Autodesk Inventor part; units mm, degrees
ref_plane "YZ Plane" through (0, 0, 0) normal (1, 0, 0) x (0, 1, 0)
ref_plane "XZ Plane" through (0, 0, 0) normal (0, 1, 0) x (-1, 0, 0)
ref_plane "XY Plane" through (0, 0, 0) normal (0, 0, 1) x (1, 0, 0)
sketch "Sketch1" plane through (0, 0, 0) normal (0, 1, 0) x (-1, 0, 0)
  line L0 (0, 0) -> (-25, 0)
  line L1 (-25, 0) -> (-25, -14)
  line L2 (-25, -14) -> (0, -14)
  line L3 (0, -14) -> (0, 0)
  dimension "d0" = 25
  dimension "d1" = 14
extrude "Extrusion1" add sketch "Sketch1" along normal blind 14
sketch "Sketch2" plane through (0, 14, 0) normal (0, 1, 0) x (1, 0, 0)
  line L0 (3.25, 4) -> (21.75, 4)
  line L1 (21.75, 4) -> (21.75, 6.4)
  line L2 (21.75, 6.4) -> (3.25, 6.4)
  line L3 (3.25, 6.4) -> (3.25, 4)
  point P0 (0, 0)
  dimension "d6" = 18.5
  dimension "d7" = 2.4
extrude "Extrusion2" cut sketch "Sketch2" against normal blind 10.3
properties part number "ServoOverServo"
The model under review builds one solid part; all positions refer to its coordinate system, in mm. A direction names the side the tool comes from. Round coordinates to 2 decimals unless told otherwise and drop trailing zeros. Order: outer loops, then holes, each group sorted by start corner. A loop starts at its lowest first (then second) coordinate and runs counter-clockwise, first axis right, second up. Notation, with made-up numbers: M 37.25,-12 L 50.25,-12 A22 ccw 50.25,23 Z; hole C -25,-8.5 d1. An arc over 180 degrees is marked long. Use a Markdown table: item, result.
1) Wall thickness on line 1 along Z through (x, y) = (8.5, 9.75); line 2 along X through (y, z) = (4.25, -5.5); line 3 along Y through (x, z) = (21, -4.75): over which ranges is each line inside the solid? List them lowest first. Write a range as [from, to].
Report:
| item | result |
|---|---|
| line 1 | [-14, -6.4], [-4, 0] |
| line 2 | [0, 3.25], [21.75, 25] |
| line 3 | [0, 3.7] |
2) Consider section B-B (x = 16.75). Write out the cut boundary in (y, z), then the cut area to 3 significant figures.
Report:
| item | result |
|---|---|
| outline | M 0,-14 L 14,-14 L 14,-6.4 L 3.7,-6.4 L 3.7,-4 L 14,-4 L 14,0 L 0,0 Z |
| area | 171 mm^2 |
3) Consider section A-A (y = 5.75). Write out the cut boundary in (x, z), then the cut area to 3 significant figures.
Report:
| item | result |
|---|---|
| outline | M 0,-14 L 25,-14 L 25,0 L 0,0 Z; hole M 3.25,-6.4 L 21.75,-6.4 L 21.75,-4 L 3.25,-4 Z |
| area | 306 mm^2 |
4) Insertion check: pin 1 (1.9 mm diameter, centred on x = 12.5, z = -5, fed in from +Y). The pin has a flat end and moves straight along its axis. Give the tip position at first contact, or say it passes through.
Report:
| item | result |
|---|---|
| pin 1 | y = 3.7 |
5) Tool access review of faces 5 (the face through (3.25, 9, -5)), 6 (the face through (13, 14, -7)): name each direction out of +Z, -Z, +X, -X, +Y, -Y from which nothing blocks a thin tool from reaching the whole face with its end or side.
Report:
| item | result |
|---|---|
| face 5 | +Y |
| face 6 | +Z, -Z, +X, -X, +Y |
6) Draft analysis for pull direction Z (two halves, no side actions). For faces 1 (the face through (12, 7, 0)), 2 (the face through (12, 9, -4)), 3 (the face through (12, 3.7, -5)), 4 (the face through (13, 7, -14)), state which applies: released by +Z, released by -Z, zero draft, split by the parting line, or undercut.
Report:
| item | result |
|---|---|
| face 1 | released by +Z |
| face 2 | undercut |
| face 3 | undercut |
| face 4 | released by -Z |
